```python
from build123d import *

# Parameters (mm, degrees)
ESQUISSE1_W             = 20
ESQUISSE1_H             = 20
BOSS_EXTRU_1_DEPTH      = 20
ENL_V_START             = -3
ESQUISSE2_R             = 2.6
ENL_V_MAT_EXTRU_1_DEPTH = 53.506491459
ENL_V_MAT_EXTRU_1_TAPER = 2
ESQUISSE3_W             = 16
ESQUISSE3_H             = 16
ENL_V_MAT_EXTRU_2_DEPTH = 18
CHANFREIN1_SIZE         = 1


with BuildPart() as part:
    # Esquisse1 → Boss.-Extru.1 (new body)
    with BuildSketch(Plane.XY):
        with Locations((-24.630410255, 19.182655502)):
            Rectangle(ESQUISSE1_W, ESQUISSE1_H)
    extrude(amount=BOSS_EXTRU_1_DEPTH)

    # Esquisse2 → Enlèv. mat.-Extru.1 (cut, through all)
    with BuildSketch(Plane.XY.offset(20).offset(ENL_V_START)):
        with Locations((-24.630410255, 19.182655502)):
            Circle(ESQUISSE2_R)
    extrude(amount=ENL_V_MAT_EXTRU_1_DEPTH, taper=ENL_V_MAT_EXTRU_1_TAPER, mode=Mode.SUBTRACT)

    # Esquisse3 → Enlèv. mat.-Extru.2 (cut)
    with BuildSketch(Plane(origin=(0, 0, 0), x_dir=(-1, 0, 0), z_dir=(0, 0, -1))):
        with Locations((24.630410255, 19.182655502)):
            Rectangle(ESQUISSE3_W, ESQUISSE3_H)
    extrude(amount=-ENL_V_MAT_EXTRU_2_DEPTH, mode=Mode.SUBTRACT)

    # Chanfrein1
    chanfrein1_edges = [part.edges().sort_by_distance(p)[0] for p in [
        (-34.630410255, 29.182655502, 10),
        (-14.630410255, 29.182655502, 10),
        (-14.630410255, 9.182655502, 10),
        (-34.630410255, 9.182655502, 10),
    ]]
    chamfer(chanfrein1_edges, length=CHANFREIN1_SIZE)


solid = part.part
```
CAD build for the part. Positions are in the model's coordinates, mm. A direction names the side the tool comes from. Round coordinates to 2 decimals unless told otherwise and drop trailing zeros. Order: outer loops, then holes, each group sorted by start corner. A loop starts at its lowest first (then second) coordinate and runs counter-clockwise, first axis right, second up. Notation, with made-up numbers: (43.25, -33.5) - (81.25, -33.5) arc R24 ccw to (81.25, -17.5) - close; hole circle Ø7 at (69, 11.5). An arc over 180 degrees is marked (long way). Use CSV: the item, a comma, the result in double quotes. Start each with the question number.
1) Pin check, flat tip, straight feed: pin 1 Ø2 at (x, y) = (-18, 21) entering from -Z. Stop position of the tip, or through.
2) Two-plate mould, pull along Y, no slides. Class faces 1 (the flat face through (-25, 9.183, 10)), 2 (the flat face through (-25, 29.183, 10)), 3 (the flat face through (-34.63, 19, 10)), 4 (the flat face through (-22.7, 21.1, 18)): pulls with the +Y half, pulls with the -Y half, needs draft (parallel to the pull), parting line crosses it, or undercut.
3) Saw through at B-B (x = -21.25). List the corners of the cut face in (y, z), and give its area (3 significant figures).
4) Saw through at A-A (z = 9.75). List the corners of the cut face in (x, y), and give its area (3 significant figures).
5) Saw through at C-C (y = 14.5). List the corners of the cut face in (x, z).
6) Wall check: L1, parallel to X at y = 25.75, z = 3.5; L2, parallel to Y at x = -26, z = 3; L3, parallel to Z at x = -21.75, y = 12.25. Give the ranges that are in metal, low to high. Write a range as [from, to].
7) Tool access for faces 5 (the flat face through (-15.123, 28.676, 9.86)), 6 (the flat face through (-16.63, 19, 9)): list every direction of +Z, -Z, +X, -X, +Y, -Y with a clear straight run to the whole face (end or side of a thin tool).
Values follow:
1,pin 1,"stops at z = 18"
2,face 1,"pulls with the -Y half"
2,face 2,"pulls with the +Y half"
2,face 3,"needs draft"
2,face 4,"undercut"
3,outline,"(9.18, 0) - (11.18, 0) - (11.18, 18) - (27.18, 18) - (27.18, 0) - (29.18, 0) - (29.18, 20) - (9.18, 20) - close"
3,area,"112 mm2"
4,outline,"(-34.63, 10.18) - (-33.63, 9.18) - (-15.63, 9.18) - (-14.63, 10.18) - (-14.63, 28.18) - (-15.63, 29.18) - (-33.63, 29.18) - (-34.63, 28.18) - close; hole (-32.63, 11.18) - (-16.63, 11.18) - (-16.63, 27.18) - (-32.63, 27.18) - close"
4,area,"142 mm2"
5,outline,"(-34.63, 0) - (-32.63, 0) - (-32.63, 18) - (-16.63, 18) - (-16.63, 0) - (-14.63, 0) - (-14.63, 20) - (-34.63, 20) - close"
6,L1,"x = [-34.63, -32.63], [-16.63, -14.63]"
6,L2,"y = [9.18, 11.18], [27.18, 29.18]"
6,L3,"z = [18, 20]"
7,face 5,"+Z, -Z, +X, +Y"
7,face 6,"-Z"
